```python
from build123d import *

# Parameters (mm, degrees)
SKETCH1_R           = 5
BOSS_EXTRUDE1_DEPTH = 6.35
SKETCH2_R           = 5
BOSS_EXTRUDE2_DEPTH = 15
LPATTERN1_COUNT     = 3
LPATTERN1_PITCH     = 30
SKETCH2_4_R         = 2.5
CUT_EXTRUDE2_DEPTH  = 83.80956065


with BuildPart() as part:
    # Sketch1 → Boss-Extrude1 (new body)
    # profile 1 of 3: a face of its own
    with BuildSketch(Plane(origin=(0, 0, 0), x_dir=(1, 0, 0), z_dir=(0, 1, 0))):
        Polygon((-18.75, 0), (0, 0), (18.75, 0), (37.5, 0), (37.5, 25.4), (-37.5, 25.4), (-37.5, 0), align=None)
        with Locations(Location((-15.279173033, 10.349093201, 0), (0, 0, 270))):
            Circle(SKETCH1_R, mode=Mode.SUBTRACT)
        with Locations(Location((18.543836974, 12.56035891, 0), (0, 0, 270))):
            Circle(SKETCH1_R, mode=Mode.SUBTRACT)
    # profile 2 of 3: a face of its own
    with BuildSketch(Plane(origin=(0, 0, 0), x_dir=(1, 0, 0), z_dir=(0, 1, 0))):
        with BuildLine():
            Line((0, -7.7), (0, 0))
            Line((0, 0), (-18.75, 0))
            Line((-18.75, 0), (-37.5, 0))
            Line((-37.5, 0), (-37.5, -25.4))
            Line((-37.5, -25.4), (0, -25.4))
            Line((0, -25.4), (0, -17.7))
            ThreePointArc((0, -17.7), (-5, -12.7), (0, -7.7))
        make_face()
    # profile 3 of 3: a face of its own
    with BuildSketch(Plane(origin=(0, 0, 0), x_dir=(1, 0, 0), z_dir=(0, 1, 0))):
        with BuildLine():
            Line((18.75, 0), (0, 0))
            Line((0, 0), (0, -7.7))
            ThreePointArc((0, -7.7), (3.535533906, -9.164466094), (5, -12.7))
            ThreePointArc((5, -12.7), (3.535533906, -16.235533906), (0, -17.7))
            Line((0, -17.7), (0, -25.4))
            Line((0, -25.4), (37.5, -25.4))
            Line((37.5, -25.4), (37.5, 0))
            Line((37.5, 0), (18.75, 0))
        make_face()
    extrude(amount=BOSS_EXTRUDE1_DEPTH)

    # Sketch2 → Boss-Extrude2 (add)
    with BuildSketch(Plane.ZY.offset(37.5)):
        with Locations((-27.448482339, 8.398482339)):
            Circle(SKETCH2_R)
    boss_extrude2 = extrude(amount=-BOSS_EXTRUDE2_DEPTH)

    # LPattern1: Boss-Extrude2 ×3
    with Locations(*[(i * LPATTERN1_PITCH, 0, 0) for i in range(1, LPATTERN1_COUNT)]):
        add(boss_extrude2)

    # Sketch2_4 → Cut-Extrude2 (cut, through all)
    with BuildSketch(Plane.ZY.offset(37.5)):
        with Locations((-27.448482339, 8.398482339)):
            Circle(SKETCH2_4_R)
    extrude(amount=-CUT_EXTRUDE2_DEPTH, mode=Mode.SUBTRACT)


solid = part.part
```
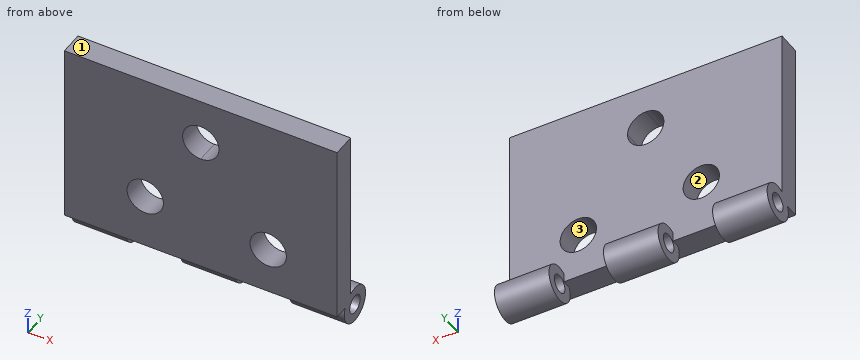
Here's how the part is built. I have some questions about the finished solid (model axes, mm). Face numbers are marked on the shaded views. Coordinates: 2 decimals unless noted, no trailing zeros. Order: outer loops, then holes, each group sorted by start corner. A loop starts at its lowest first (then second) coordinate and runs counter-clockwise, first axis right, second up.
1) We'd pull the mould along X, two halves only. Please class the marked faces 1, 2 and 3: +X half, -X half, draft (parallel to the pull), parting line (faces both ways), or undercut.
2) I need wall thicknesses on line 1 (Z direction, x = 28.5, y = 8.5); line 2 (Y direction, x = -28.5, z = 20); line 3 (Z direction, x = -16, y = 1). Which ranges of each line are inside material? Lowest first, please.
3) Imagine slicing it at B-B on y = 4.75. List the corners of the cut face in (x, z) for me.
4) Imagine slicing it at A-A on x = 19.5. List the corners of the cut face in (y, z) for me.
5) Imagine slicing it at C-C on x = -6.5. List the corners of the cut face in (y, z) for me, and give its area (3 significant figures).
6) Will these pins go through, and if not, where does the flat tip stop? pin 1 (1 mm diameter, centred on x = -25, z = -9.5, fed in from +Y); pin 2 (2 mm diameter, centred on x = 24.5, y = 5.5, fed in from -Z).
Response values:
1. face 1: draft
1. face 2: undercut
1. face 3: undercut
2. line 1: z = -32.45 to -29.95, -24.95 to -22.45
2. line 2: y = 0 to 6.35
2. line 3: z = -25.4 to -15.3, -5.4 to 25.4
3. outline: (-37.5, -30.87) - (-22.5, -30.87) - (-22.5, -25.4) - (-7.5, -25.4) - (-7.5, -30.87) - (7.5, -30.87) - (7.5, -25.4) - (22.5, -25.4) - (22.5, -30.87) - (37.5, -30.87) - (37.5, 25.4) - (-37.5, 25.4) - close; hole circle Ø10 at (-15.28, -10.35); hole circle Ø10 at (0, 12.7); hole circle Ø10 at (18.54, -12.56)
4. outline: (0, -25.4) - (6.35, -25.4) - (6.35, -17.47) - (0, -17.47) - close; (0, -7.65) - (6.35, -7.65) - (6.35, 25.4) - (0, 25.4) - close
5. outline: (0, -25.4) - (3.84, -25.4) arc R5 ccw (long way) to (6.35, -22.89) - (6.35, 25.4) - (0, 25.4) - close; hole circle Ø5 at (8.4, -27.45)
5. area: 378 mm2
6. pin 1: stops at y = 6.35
6. pin 2: stops at z = -32.07
